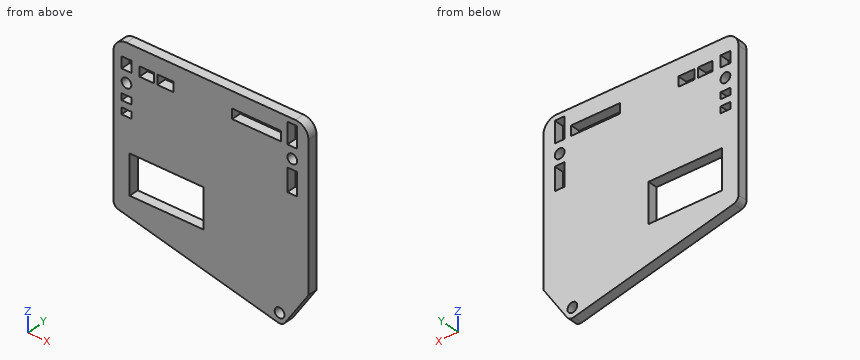
from build123d import *

# Parameters (mm, degrees)
CROQUIS1_R                 = 1.5
CROQUIS1_W                 = 3
CROQUIS1_H                 = 6.464673287
CROQUIS1_W_2               = 3.020034148
CROQUIS1_H_2               = 3.461191377
CROQUIS1_W_3               = 4.5
CROQUIS1_H_3               = 2.964673291
CROQUIS1_W_4               = 5
CROQUIS1_W_5               = 15
CROQUIS1_H_4               = 3
CROQUIS1_H_5               = 7
CROQUIS1_W_6               = 3.007385003
CROQUIS1_H_6               = 1.999998024
CROQUIS1_W_7               = 3.001763161
CROQUIS1_H_7               = 1.995781642
CROQUIS1_W_8               = 22.700000001
CROQUIS1_H_8               = 12
SALIENTE_EXTRUIR1_DEPTH    = 3
S_LIDO_MOVER_COPIAR1_ANGLE = 90


with BuildPart() as part:
    # Croquis1 → Saliente-Extruir1 (new body)
    with BuildSketch(Plane.XY):
        with BuildLine():
            Line((41808.502638122, -312.734450912), (41808.502638122, -355.143425671))
            ThreePointArc((41808.502638122, -355.143425671), (41808.937480298, -356.388528473), (41810.052919108, -357.092208062))
            Line((41810.052919108, -357.092208062), (41859.155637399, -368.423604591))
            ThreePointArc((41859.155637399, -368.423604591), (41860.343476449, -368.333633328), (41861.269457002, -367.584222592))
            Line((41861.269457002, -367.584222592), (41868.502638122, -356.734450911))
            Line((41868.502638122, -356.734450911), (41868.502638122, -312.734450912))
            ThreePointArc((41868.502638122, -312.734450912), (41867.331065246, -309.906023787), (41864.502638122, -308.734450912))
            Line((41864.502638122, -308.734450912), (41812.502638122, -308.734450912))
            ThreePointArc((41812.502638122, -308.734450912), (41809.674210997, -309.906023787), (41808.502638122, -312.734450912))
        make_face()
        with Locations((41859.605356413, -365.4748222)):
            Circle(CROQUIS1_R, mode=Mode.SUBTRACT)
        with Locations((41812.517756121, -320.195638832)):
            Circle(CROQUIS1_R, mode=Mode.SUBTRACT)
        with Locations((41863.502638122, -320.199124199)):
            Circle(CROQUIS1_R, mode=Mode.SUBTRACT)
        with Locations((41863.502638122, -313.466787555)):
            Rectangle(CROQUIS1_W, CROQUIS1_H, mode=Mode.SUBTRACT)
        with Locations((41812.512655196, -314.965046601)):
            Rectangle(CROQUIS1_W_2, CROQUIS1_H_2, mode=Mode.SUBTRACT)
        with Locations((41818.752638122, -315.216787557)):
            Rectangle(CROQUIS1_W_3, CROQUIS1_H_3, mode=Mode.SUBTRACT)
        with Locations((41824.502638122, -315.216787557)):
            Rectangle(CROQUIS1_W_4, CROQUIS1_H_3, mode=Mode.SUBTRACT)
        with Locations((41852.502638122, -315.199124203)):
            Rectangle(CROQUIS1_W_5, CROQUIS1_H_4, mode=Mode.SUBTRACT)
        with Locations((41863.502638122, -326.734450912)):
            Rectangle(CROQUIS1_W, CROQUIS1_H_5, mode=Mode.SUBTRACT)
        with Locations((41812.506330624, -324.695634388)):
            Rectangle(CROQUIS1_W_6, CROQUIS1_H_6, mode=Mode.SUBTRACT)
        with Locations((41812.503519702, -328.697738628)):
            Rectangle(CROQUIS1_W_7, CROQUIS1_H_7, mode=Mode.SUBTRACT)
        with Locations((41824.852638123, -345.734450912)):
            Rectangle(CROQUIS1_W_8, CROQUIS1_H_8, mode=Mode.SUBTRACT)
    extrude(amount=SALIENTE_EXTRUIR1_DEPTH)


with BuildPart() as part_1:
    # Sólido-Mover/Copiar1: moved
    add(part.part.rotate(Axis((0, -338.604636556, 1.5), (1, 0, 0)), S_LIDO_MOVER_COPIAR1_ANGLE))


solid = part_1.part
Here's how the part is built. I have some questions about the finished solid (model axes, mm). Round coordinates to 2 decimals unless told otherwise and drop trailing zeros. Order: outer loops, then holes, each group sorted by start corner. A loop starts at its lowest first (then second) coordinate and runs counter-clockwise, first axis right, second up. Notation, with made-up numbers: (34.25, 81.25) -> (56.25, 81.25) arc R17 ccw to (56.25, 95.25) -> close; hole circle Ø10 at (-25, 15.5). An arc over 180 degrees is marked (long way). Use CSV: the item, a comma, the result in double quotes.
1. I want a section at B-B on x = 41855.5. List the corners of the cut face in (y, z) for me.
Recorded:
outline,"(-340.1, -27.48) -> (-337.1, -27.48) -> (-337.1, 23.41) -> (-340.1, 23.41) -> close; (-340.1, 26.41) -> (-337.1, 26.41) -> (-337.1, 31.37) -> (-340.1, 31.37) -> close"
2. I need wall thicknesses on line 1 along X through (y, z) = (-337.15, 15.5); line 2 along X through (y, z) = (-338.5, 13); line 3 along Z through (x, y) = (41818, -337.35). Which ranges of each line are inside material? Lowest first, please.
Recorded:
line 1,"x = 41808.5 to 41811, 41814.01 to 41862, 41865 to 41868.5"
line 2,"x = 41808.5 to 41862, 41865 to 41868.5"
line 3,"z = -18.82 to -11.63, 0.37 to 23.41, 26.37 to 31.37"
3. I want a section at A-A on z = -5.5. List the corners of the cut face in (x, y) for me, and give its area (3 significant figures).
Recorded:
outline,"(41808.5, -340.1) -> (41813.5, -340.1) -> (41813.5, -337.1) -> (41808.5, -337.1) -> close; (41836.2, -340.1) -> (41868.5, -340.1) -> (41868.5, -337.1) -> (41836.2, -337.1) -> close"
area,"112 mm2"
4. I'm going to push flat-ended pins straight in: P1, Ø1.5, axis at x = 41827.5, z = -11, coming from the +Y side; P2, Ø1, axis at y = -338.5, z = -21, coming from the +X side. Where does each tip first touch, or does it pass through?
Recorded:
P1,"stops at y = -337.1"
P2,"stops at x = 41865.92"
5. I want a section at C-C on y = -338.6. Give the number of separate pieces and of enclosed holes in the cut face, and give its area (3 significant figures).
Recorded:
separate pieces,"1"
enclosed holes,"12"
area,"2,800 mm2"
6. I want a section at D-D on x = 41837. List the corners of the cut face in (y, z) for me, and give its area (3 significant figures).
Recorded:
outline,"(-340.1, -23.21) -> (-337.1, -23.21) -> (-337.1, 31.37) -> (-340.1, 31.37) -> close"
area,"164 mm2"
